The figure shows three views and two pictorial views of one solid part (mm, origin at its lowest corner). Answer the questions. Give positions to 0.01 mm unless a question says otherwise; leave off trailing zeros. Loops run counter-clockwise (first coordinate to the right, second up) from the corner with the lowest first, then second, coordinate; pieces in that order, holes last. Notation, with made-up numbers: (-22, -37) - (24, -37) arc R26 ccw to (24, -20) - close; hole circle Ø3 at (78.25, 40.5). An arc over 180 degrees is marked (long way). Use a Markdown table: item, result. Add a question column.
Item 1: Consider probe 1 along X at (y, z) = (27.5, 76.5); probe 2 along Z at (x, y) = (133.35, 32.5); probe 3 along Z at (x, y) = (131, 47.5). Determine where each line is inside the solid, lowest interval first. Write a range as [from, to].
Item 2: For a pull along Z with two mould halves and no side action, classify the marked faces 1, 2 and 3 as +Z half, -Z half, draft (parallel to the pull), parting line (faces both ways), or undercut.
Item 3: A cutting plane is placed at D-D (x = 132.5). Determine the outline of the cut face in (y, z).
Item 4: A cutting plane is placed at C-C (y = 34.5). Determine the outline of the cut face in (x, z).
Item 5: A cutting plane is placed at B-B (x = 196.85). Determine the outline of the cut face in (y, z), plus the area to 3 significant figures.
Item 6: A cutting plane is placed at A-A (z = 76.2). Determine the outline of the cut face in (x, y).
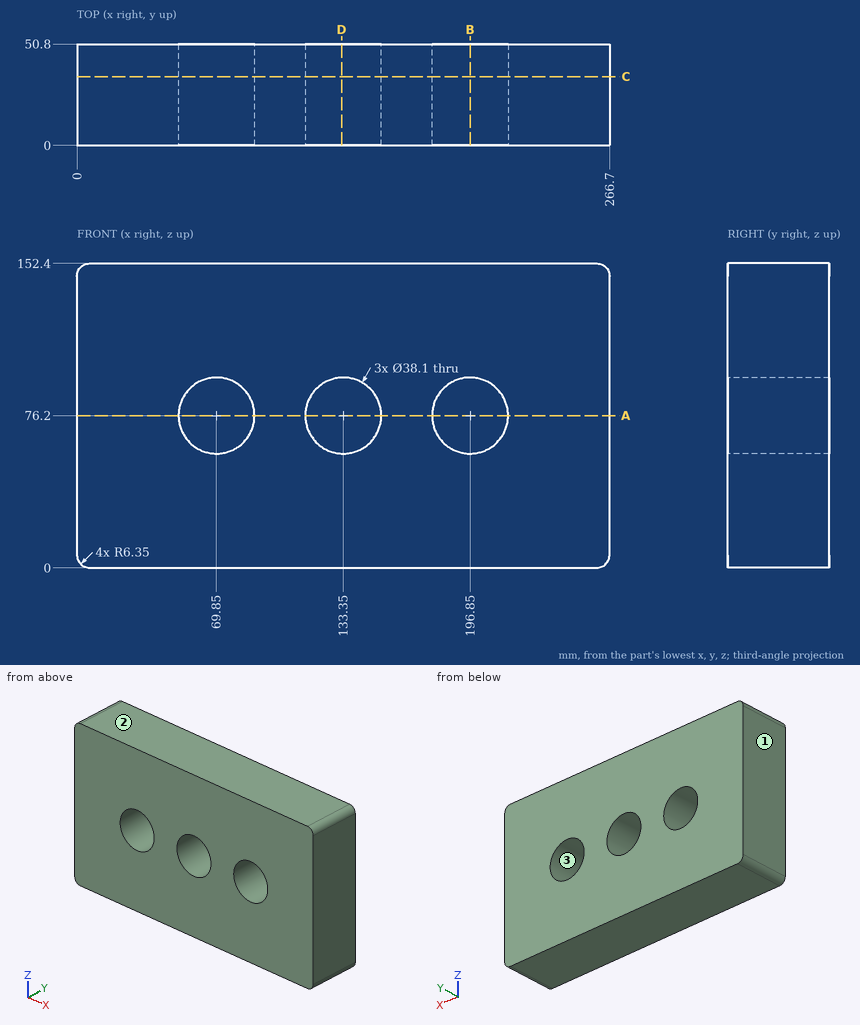
Geometry says:
| question | item | result |
|---|---|---|
| 1 | probe 1 | [0, 50.8], [88.9, 114.3], [152.4, 177.8], [215.9, 266.7] |
| 1 | probe 2 | [0, 57.15], [95.25, 152.4] |
| 1 | probe 3 | [0, 57.3], [95.1, 152.4] |
| 2 | face 1 | draft |
| 2 | face 2 | +Z half |
| 2 | face 3 | undercut |
| 3 | outline | (0, 0) - (50.8, 0) - (50.8, 57.17) - (0, 57.17) - close; (0, 95.23) - (50.8, 95.23) - (50.8, 152.4) - (0, 152.4) - close |
| 4 | outline | (0, 6.35) arc R6.35 ccw to (6.35, 0) - (260.35, 0) arc R6.35 ccw to (266.7, 6.35) - (266.7, 146.05) arc R6.35 ccw to (260.35, 152.4) - (6.35, 152.4) arc R6.35 ccw to (0, 146.05) - close; hole circle Ø38.1 at (69.85, 76.2); hole circle Ø38.1 at (133.35, 76.2); hole circle Ø38.1 at (196.85, 76.2) |
| 5 | outline | (0, 0) - (50.8, 0) - (50.8, 57.15) - (0, 57.15) - close; (0, 95.25) - (50.8, 95.25) - (50.8, 152.4) - (0, 152.4) - close |
| 5 | area | 5,810 mm² |
| 6 | outline | (0, 0) - (50.8, 0) - (50.8, 50.8) - (0, 50.8) - close; (88.9, 0) - (114.3, 0) - (114.3, 50.8) - (88.9, 50.8) - close; (152.4, 0) - (177.8, 0) - (177.8, 50.8) - (152.4, 50.8) - close; (215.9, 0) - (266.7, 0) - (266.7, 50.8) - (215.9, 50.8) - close |
